Verification items for this drawing (mm, ordinates from the low corner). A direction names the side the tool comes from. Coordinates: 2 decimals unless noted, no trailing zeros. Loops run counter-clockwise (first coordinate to the right, second up) from the corner with the lowest first, then second, coordinate; pieces in that order, holes last. Notation, with made-up numbers: M 20.25,-15.5 L 45.25,-15.5 A6 ccw 45.25,-5.5 Z; hole C 82,-29.75 d3. An arc over 180 degrees is marked long. Return JSON: item names as keys, results as strings.
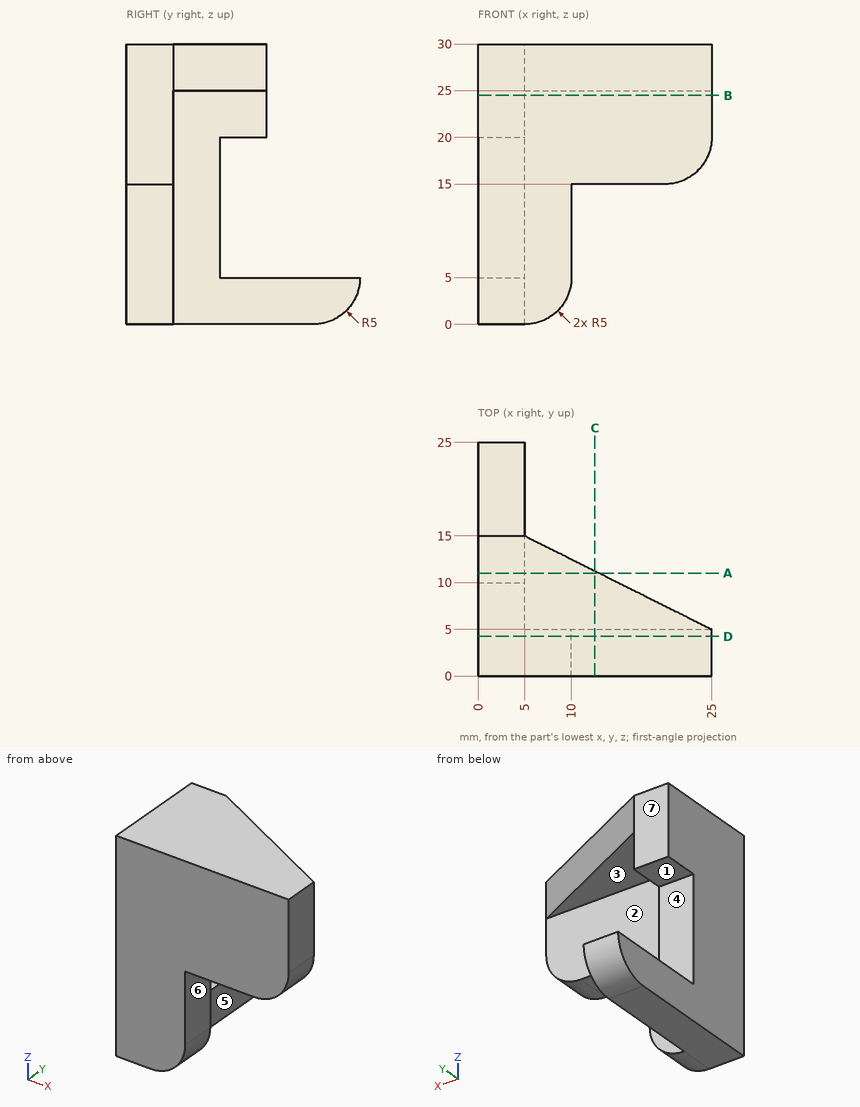
1) Section check A-A on y = 11. Record the cut outline in (x, z), then the cut area to 3 significant figures.
Answers:
{"outline": "M 0,0 L 5,0 L 5,5 L 0,5 Z; M 0,20 L 5,20 L 5,25 L 13,25 L 13,30 L 0,30 Z", "area": "115 mm²"}
2) Section check C-C on x = 12.5. Record the cut outline in (y, z).
Answers:
{"outline": "M 0,15 L 5,15 L 5,25 L 11.25,25 L 11.25,30 L 0,30 Z"}
3) Section check B-B on z = 24.5. Record the cut outline in (x, y).
Answers:
{"outline": "M 0,0 L 25,0 L 25,5 L 5,5 L 5,15 L 0,15 Z"}
4) Scan lines: line 1 along Z through (x, y) = (2, 13.5); line 2 along Y through (x, z) = (7.5, 19). Record each from-to range of solid material in increasing order. Write a range as [from, to].
Answers:
{"line 1": "[0, 5], [20, 30]", "line 2": "[0, 5]"}
5) Section check D-D on y = 4.25. Record the cut outline in (x, z).
Answers:
{"outline": "M 0,0 L 5,0 A5 ccw 10,5 L 10,15 L 20,15 A5 ccw 25,20 L 25,30 L 0,30 Z"}
6) Go/stop test with flat-tipped pins: pin 1 Ø5.5 at (x, y) = (17.5, 3.5) entering from -Z; pin 2 Ø3 at (x, y) = (20, 7.5) entering from -Z; pin 3 Ø1.5 at (x, z) = (2, 11) entering from +Y. Record where each tip stops, or that it passes through.
Answers:
{"pin 1": "z = 15", "pin 2": "z = 25", "pin 3": "y = 10"}
7) Set-up check for the marked faces 4, 5, 6 and 7: record each of +Z, -Z, +X, -X, +Y, -Y from which the full face is reachable in a straight line by a thin tool's end or side.
Answers:
{"face 4": "+X, -X, +Y", "face 5": "-Z, +X, +Y", "face 6": "-Z, +X, +Y, -Y", "face 7": "+Z, +X, -X, +Y"}
8) Draft check along Z on the marked faces 1, 2 and 3. Enter one of: +Z half, -Z half, draft (parallel to the pull), parting line (faces both ways), or undercut.
Answers:
{"face 1": "undercut", "face 2": "draft", "face 3": "-Z half"}
